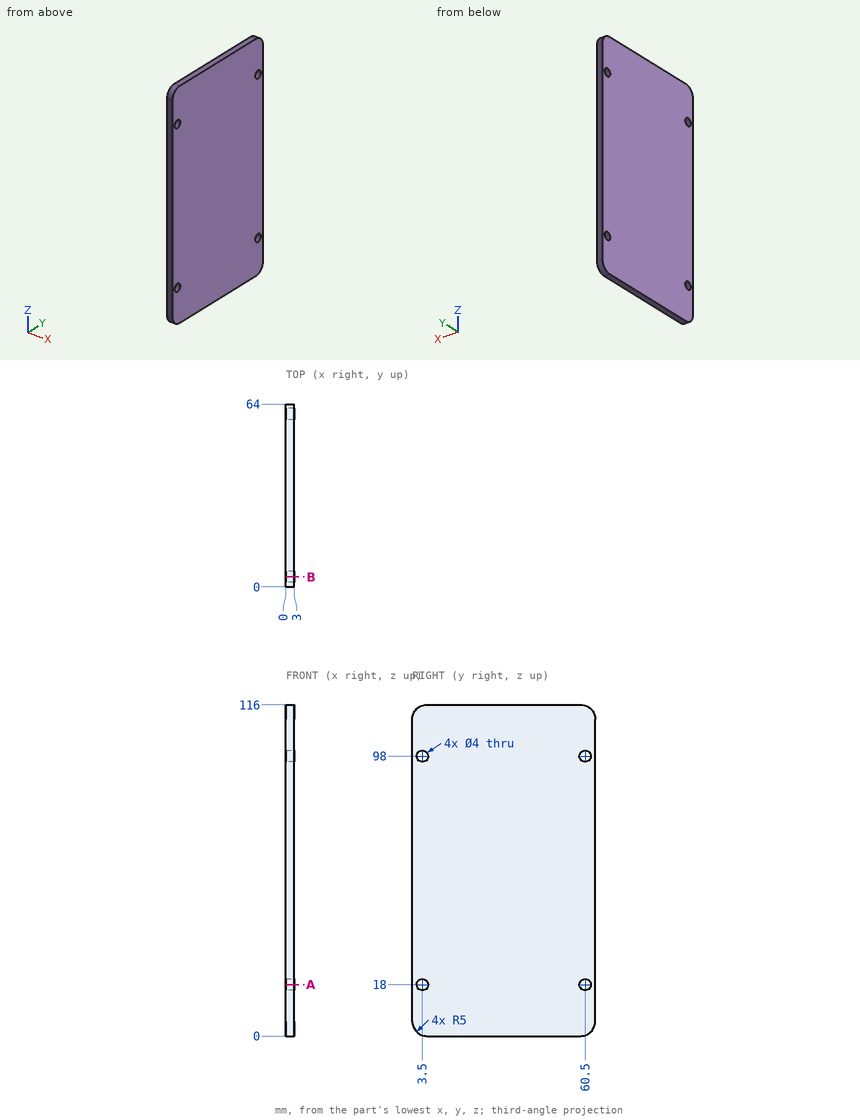
For this review, use the dimensioned drawing (mm, ordinates from the lowest corner) and the shaded views. Coordinates: 2 decimals unless noted, no trailing zeros. Order: outer loops, then holes, each group sorted by start corner. A loop starts at its lowest first (then second) coordinate and runs counter-clockwise, first axis right, second up. Notation, with made-up numbers: (12.25, 65) - (26.25, 65) arc R8 ccw to (26.25, 70) - close; hole circle Ø1 at (-20, -13). An arc over 180 degrees is marked (long way). Use one line per item in the form item = value.
Q1. Consider section A-A (z = 18). Give the boundary of the cut face in (x, y), then the cut area to 3 significant figures.
Checked values:
outline = (0, 0) - (3, 0) - (3, 1.5) - (0, 1.5) - close; (0, 5.5) - (3, 5.5) - (3, 58.5) - (0, 58.5) - close; (0, 62.5) - (3, 62.5) - (3, 64) - (0, 64) - close
area = 168 mm2
Q2. For P1, Ø3.5, axis at y = 3.5, z = 18, coming from the +X side, flat-tipped, find the tip position at first contact; note if it passes through.
Checked values:
P1 = through
Q3. For probe 1 along Y at (x, z) = (1.2, 98); probe 2 along Y at (x, z) = (1.1, 97); probe 3 along Z at (x, y) = (1.55, 5), list the stretches that pass through material, from the lowest coordinate up. Write a range as from..to.
Checked values:
probe_1 = 0..1.5, 5.5..58.5, 62.5..64
probe_2 = 0..1.77, 5.23..58.77, 62.23..64
probe_3 = 0..16.68, 19.32..96.68, 99.32..116
Q4. Consider section B-B (y = 3.5). Give the boundary of the cut face in (x, z).
Checked values:
outline = (0, 0.23) - (3, 0.23) - (3, 16) - (0, 16) - close; (0, 20) - (3, 20) - (3, 96) - (0, 96) - close; (0, 100) - (3, 100) - (3, 115.77) - (0, 115.77) - close
